Autodesk Inventor part; units mm, degrees
ref_plane "YZ Plane" through (0, 0, 0) normal (1, 0, 0) x (0, 1, 0)
ref_plane "XZ Plane" through (0, 0, 0) normal (0, 1, 0) x (-1, 0, 0)
ref_plane "XY Plane" through (0, 0, 0) normal (0, 0, 1) x (1, 0, 0)
sketch "Sketch1" plane through (0, 0, 0) normal (0, 1, 0) x (-1, 0, 0)
  circle A0 centre (28.1298, -0.9274) radius 1
  circle A1 centre (3.1298, -25.9274) radius 1
  circle A2 centre (-21.8702, -0.9274) radius 1
  circle A3 centre (3.1298, 24.0726) radius 1
  line L0 (33.1298, -30.9274) -> (-26.8702, -30.9274)
  line L1 (-26.8702, -30.9274) -> (-26.8702, 29.0726)
  line L2 (-26.8702, 29.0726) -> (33.1298, 29.0726)
  line L3 (33.1298, 29.0726) -> (33.1298, -30.9274)
  line L4 (33.1298, -30.9274) -> (-26.8702, 29.0726) construction
  line L5 (-26.8702, -30.9274) -> (33.1298, 29.0726) construction
  point P0 (0, 0)
  dimension "d1" = 2
  dimension "d2" = 2
  dimension "d3" = 2
  dimension "d4" = 2
  dimension "d7" = 60
  dimension "d9" = 50
  dimension "d10" = 50
  dimension "d12" = 5
  dimension "d13" = 60
  dimension "d14" = 5
  dimension "d15" = 30
  dimension "d16" = 30
  dimension "d17" = 30
extrude "Extrusion1" add sketch "Sketch1" along normal blind 5 contours A0 | A1 | A2 | A3 | L0 L1 L2 L3
sketch "Sketch2" plane through (0, 5, 0) normal (0, 1, 0) x (1, 0, 0)
  line L0 (26.8702, 30.9274) -> (-33.1298, 30.9274)
  line L1 (-7.7791, 30.9274) -> (2.2209, 30.9274)
  line L2 (2.2209, 30.9274) -> (2.2209, 40.9274)
  line L3 (2.2209, 40.9274) -> (-7.7791, 40.9274)
  line L4 (-7.7791, 40.9274) -> (-7.7791, 30.9274)
  line L5 (-33.1298, -29.0726) -> (26.8702, -29.0726)
  line L6 (-7.7791, -29.0726) -> (2.2209, -29.0726)
  line L7 (2.2209, -29.0726) -> (2.2209, -39.0726)
  line L8 (2.2209, -39.0726) -> (-7.7791, -39.0726)
  line L9 (-7.7791, -39.0726) -> (-7.7791, -29.0726)
  point P0 (0, 0)
  dimension "d18" = 10
  dimension "d19" = 10
  dimension "d20" = 10
extrude "Extrusion2" add sketch "Sketch2" against normal blind 5
sketch "Sketch3" plane through (0, 0, 0) normal (0, -1, 0) x (1, 0, 0)
  circle A0 centre (-2.7791, -36.9274) radius 2.925
  circle A1 centre (-2.7791, 35.0726) radius 2.925
  line L0 (-7.7791, 39.0726) -> (-7.7791, 29.0726)
  line L1 (2.2209, 39.0726) -> (-7.7791, 39.0726)
  line L2 (-7.7791, -40.9274) -> (2.2209, -40.9274)
  line L3 (-7.7791, -30.9274) -> (-7.7791, -40.9274)
  point P0 (0, 0)
  dimension "d23" = 5.85
  dimension "d24" = 5.85
  dimension "d25" = 5
  dimension "d26" = 4
  dimension "d27" = 4
  dimension "d28" = 5
extrude "Extrusion3" cut sketch "Sketch3" along normal through all both and the other way through all
sketch "Sketch4" plane through (0, 0, 0) normal (0, -1, 0) x (1, 0, 0)
  line L0 (-10.1298, 6.0726) -> (3.8702, 6.0726)
  line L1 (3.8702, 6.0726) -> (3.8702, -7.9274)
  line L2 (3.8702, -7.9274) -> (-10.1298, -7.9274)
  line L3 (-10.1298, -7.9274) -> (-10.1298, 6.0726)
  line L4 (-33.1298, 29.0726) -> (-33.1298, -30.9274)
  line L5 (26.8702, -30.9274) -> (26.8702, 29.0726)
  line L6 (-33.1298, -30.9274) -> (-7.7791, -30.9274)
  line L7 (26.8702, 29.0726) -> (-33.1298, 29.0726)
  point P0 (0, 0)
  point P1 (-7.7791, 29.0726)
  dimension "d31" = 14
  dimension "d32" = 14
  dimension "d33" = 23
  dimension "d34" = 23
  dimension "d35" = 23
  dimension "d36" = 23
extrude "Extrusion4" cut sketch "Sketch4" against normal through all
sketch "Sketch5" plane through (0, 5, 0) normal (0, 1, 0) x (1, 0, 0)
  line L0 (-43.1298, -4.0726) -> (-33.1298, -4.0726)
  line L1 (-33.1298, -4.0726) -> (-33.1298, 5.9274)
  line L2 (-33.1298, 5.9274) -> (-43.1298, 5.9274)
  line L3 (-43.1298, 5.9274) -> (-43.1298, -4.0726)
  line L4 (-33.1298, -29.0726) -> (-7.7791, -29.0726)
  line L5 (-33.1298, 30.9274) -> (-33.1298, -29.0726)
  line L6 (26.8702, 30.9274) -> (26.8702, -29.0726)
  line L7 (26.8702, -4.0726) -> (36.8702, -4.0726)
  line L8 (36.8702, -4.0726) -> (36.8702, 5.9274)
  line L9 (36.8702, 5.9274) -> (26.8702, 5.9274)
  line L10 (26.8702, 5.9274) -> (26.8702, -4.0726)
  line L11 (26.8702, 30.9274) -> (2.2209, 30.9274)
  line L12 (2.2209, -29.0726) -> (26.8702, -29.0726)
  line L13 (26.8702, -29.0726) -> (26.8702, 30.9274)
  point P0 (0, 0)
  dimension "d39" = 10
  dimension "d40" = 10
  dimension "d41" = 25
  dimension "d42" = 0
  dimension "d43" = 10
  dimension "d44" = 10
  dimension "d45" = 25
  dimension "d46" = 25
  dimension "d47" = 10
extrude "Extrusion5" add sketch "Sketch5" against normal blind 5
sketch "Sketch6" plane through (0, 5, 0) normal (0, 1, 0) x (1, 0, 0)
  circle A0 centre (-39.1298, 0.9274) radius 2.925
  circle A1 centre (32.8702, 0.9274) radius 2.925
  line L0 (36.8702, 5.9274) -> (26.8702, 5.9274)
  line L1 (26.8702, -29.0726) -> (26.8702, -4.0726)
  line L2 (36.8702, -4.0726) -> (36.8702, 5.9274)
  line L3 (-43.1298, 5.9274) -> (-43.1298, -4.0726)
  line L4 (-33.1298, 5.9274) -> (-43.1298, 5.9274)
  point P0 (0, 0)
  dimension "d50" = 5.85
  dimension "d51" = 5.85
  dimension "d52" = 5
  dimension "d54" = 4
  dimension "d55" = 4
  dimension "d56" = 5
extrude "Extrusion6" cut sketch "Sketch6" against normal through all
sketch "Sketch7" plane through (0, 5, 0) normal (0, 1, 0) x (1, 0, 0)
  line L0 (-24.9285, -19.3498) -> (16.3215, -19.3498)
  line L1 (16.3215, -19.3498) -> (16.3215, 21.9002)
  line L2 (16.3215, 21.9002) -> (-24.9285, 21.9002)
  line L3 (-24.9285, 21.9002) -> (-24.9285, -19.3498)
  line L4 (-33.1298, -29.0726) -> (-7.7791, -29.0726)
  line L5 (26.8702, -29.0726) -> (26.8702, -4.0726)
  line L6 (-31.8035, -26.2248) -> (23.1965, -26.2248)
  line L7 (23.1965, -26.2248) -> (23.1965, 28.7752)
  line L8 (23.1965, 28.7752) -> (-31.8035, 28.7752)
  line L9 (-31.8035, 28.7752) -> (-31.8035, -26.2248)
  line L10 (26.8702, 30.9274) -> (2.2209, 30.9274)
  line L11 (2.2209, -29.0726) -> (26.8702, -29.0726)
  line L12 (-33.1298, -4.0726) -> (-33.1298, -29.0726)
  point P0 (0, 0)
  dimension "d78" = 55
extrude "Extrusion7" add sketch "Sketch7" along normal blind 6
sketch "Sketch8" plane through (0, 11, 0) normal (0, 1, 0) x (1, 0, 0)
  circle A0 centre (-27.9285, 11.9002) radius 0.75
  line L0 (-24.9285, -19.3498) -> (-24.9285, 21.9002)
  line L1 (-24.9285, 21.9002) -> (16.3215, 21.9002)
  point P0 (0, 0)
  dimension "d70" = 1.5
  dimension "d71" = 3
  dimension "d80" = 10
sketch "Sketch9" plane through (-24.9285, 5, 19.3498) normal (1, 0, 0) x (0, 0, -1)
  circle A0 centre (31.25, 2.5) radius 0.75
  line L0 (0, 6) -> (41.25, 6)
  point P0 (19.3498, -5)
  dimension "d72" = 1.5
  dimension "d73" = 3.5
  dimension "d81" = 10
loft "Loft1" cut profiles "Sketch9", "Sketch8"
sketch "Sketch10" plane through (0, 11, 0) normal (0, 1, 0) x (1, 0, 0)
  circle A0 centre (-28.4285, -12.1344) radius 1.75
  line L0 (-24.9285, -19.3498) -> (-24.9285, 21.9002)
  point P0 (0, 0)
  dimension "d83" = 3.5
  dimension "d84" = 3.5
sketch "Sketch11" plane through (-24.9285, 5, 19.3498) normal (1, 0, 0) x (0, 0, -1)
  circle A0 centre (6.8624, 3) radius 2
  line L0 (41.25, 0) -> (0, 0)
  point P0 (19.3498, -5)
  dimension "d85" = 4
  dimension "d86" = 3
loft "Loft2" cut profiles "Sketch10", "Sketch11"
sketch "Sketch13" plane through (0, 5, 0) normal (0, 1, 0) x (1, 0, 0)
  line L0 (10.8215, -14.0787) -> (-17.1785, -14.0787)
  line L1 (-17.1785, -14.0787) -> (-17.1785, 15.9213)
  line L2 (-17.1785, 15.9213) -> (10.8215, 15.9213)
  line L3 (10.8215, 15.9213) -> (10.8215, -14.0787)
  line L4 (16.3215, 21.9002) -> (16.3215, -19.3498)
  point P0 (0, 0)
  point P1 (-12.1298, -8.0726)
  point P2 (5.8702, 9.9274)
  dimension "d104" = 30
  dimension "d105" = 28
  dimension "d106" = 5.5
extrude "Extrusion9" cut sketch "Sketch13" against normal blind 2
properties part number "LidClampCell_V6"
Model file for the job. Use its own axes, mm. A direction names the side the tool comes from. Give positions to 0.01 mm unless a question says otherwise; leave off trailing zeros. Loops run counter-clockwise (first coordinate to the right, second up) from the corner with the lowest first, then second, coordinate; pieces in that order, holes last. Notation, with made-up numbers: (2, 67) - (46, 67) arc R17 ccw to (46, 98) - close; hole circle Ø6 at (-7.5, 43.5). An arc over 180 degrees is marked (long way). Use one line per item in the form item = value.
(1) Cut at C-C (z = -23). Give the cut face in (x, y).
Determined:
outline = (-33.13, 0) - (26.87, 0) - (26.87, 5) - (23.2, 5) - (23.2, 11) - (-31.8, 11) - (-31.8, 5) - (-33.13, 5) - close
(2) 3-axis set-ups, long thin cutter, end or side, ignore diameter. For faces 5 (the face through (-24.928, 8, -2)), 6 (the face through (-3, 1, -7.927)), 7 (the face through (-33.13, 2, 17)), 8 (the face through (-5, 8, 26.225)), 9 (the face through (32, 3, -5.927)): which of +Z, -Z, +X, -X, +Y, -Y reach the whole face in a straight line?
Determined:
face_5 = +Y
face_6 = +Y, -Y
face_7 = +Z, -X, +Y, -Y
face_8 = +Z, +X, -X, +Y
face_9 = -Z, +X, +Y, -Y
(3) Cut at A-A (z = -7). Give the cut face in (x, y).
Determined:
outline = (-33.13, 0) - (-10.13, 0) - (-10.13, 3) - (-17.18, 3) - (-17.18, 5) - (-24.93, 5) - (-24.93, 11) - (-31.8, 11) - (-31.8, 5) - (-33.13, 5) - close; (3.87, 0) - (26.87, 0) - (26.87, 5) - (23.2, 5) - (23.2, 11) - (16.32, 11) - (16.32, 5) - (10.82, 5) - (10.82, 3) - (3.87, 3) - close
(4) Drop flat-ended pins along their axis: P1, Ø1.5, axis at x = -31.5, y = 7, coming from the -Z side; P2, Ø5, axis at y = 5.5, z = 11, coming from the +X side; P3, Ø4, axis at y = 3, z = 14, coming from the -X side; P4, Ø3.5, axis at x = -2.78, z = -36.93, coming from the -Y side. Give the stop position or say it passes through.
Determined:
P1 = -28.78
P2 = 26.87
P3 = -33.13
P4 = through
(5) Pull direction X, two halves, no side cores. Call faces 1 (the face through (-4, 8, -21.9)), 2 (the face through (36.87, 3, -1)), 3 (the face through (30.549, 2.535, 0.852)), 4 (the face through (-21, 2, -30.927)): pulls with the +X half, pulls with the -X half, needs draft (parallel to the pull), parting line crosses it, or undercut.
Determined:
face_1 = undercut
face_2 = pulls with the +X half
face_3 = undercut
face_4 = needs draft
(6) Cut at B-B (x = 15). Give the cut face in (y, z), then the cut area to 4 significant figures.
Determined:
outline = (0, -30.93) - (5, -30.93) - (5, -28.78) - (11, -28.78) - (11, -21.9) - (5, -21.9) - (5, 19.35) - (11, 19.35) - (11, 26.22) - (5, 26.22) - (5, 29.07) - (0, 29.07) - close
area = 382.5 mm^2
(7) Cut at D-D (y = 2). Give the cut face in (x, z) (3 decimals), then the cut area to 3 significant figures.
Determined:
outline = (-43.13, -5.927) - (-33.13, -5.927) - (-33.13, -30.927) - (-7.779, -30.927) - (-7.779, -40.927) - (2.221, -40.927) - (2.221, -30.927) - (26.87, -30.927) - (26.87, -5.927) - (36.87, -5.927) - (36.87, 4.073) - (26.87, 4.073) - (26.87, 29.073) - (2.221, 29.073) - (2.221, 39.073) - (-7.779, 39.073) - (-7.779, 29.073) - (-33.13, 29.073) - (-33.13, 4.073) - (-43.13, 4.073) - close; hole circle Ø5.85 at (-39.13, -0.927); hole (-10.13, -7.927) - (3.87, -7.927) - (3.87, 6.073) - (-10.13, 6.073) - close; hole circle Ø5.85 at (-2.779, -36.927); hole circle Ø5.85 at (-2.779, 35.073); hole circle Ø5.85 at (32.87, -0.927)
area = 3,700 mm^2
(8) Drill centre lines: L1, parallel to X at y = 1, z = 35 (3 decimals); L2, parallel to X at y = 6, z = 7; L3, parallel to Z at x = 6, y = 3.5. Where is each one in solid material? Low to high.
Determined:
L1 = -7.779 to -5.703, 0.145 to 2.221
L2 = -31.8 to -24.93, 16.32 to 23.2
L3 = -30.93 to -15.92, 14.08 to 29.07
